CAD build for the part. Positions are in the model's coordinates, mm. Face numbers are marked on the shaded views. Round coordinates to 2 decimals unless told otherwise and drop trailing zeros. Order: outer loops, then holes, each group sorted by start corner. A loop starts at its lowest first (then second) coordinate and runs counter-clockwise, first axis right, second up. Notation, with made-up numbers: M -8,10.5 L 8,10.5 A11 ccw 8,25.5 Z; hole C 68.5,-24 d3. An arc over 180 degrees is marked long. Put each result on its own line as item: value.
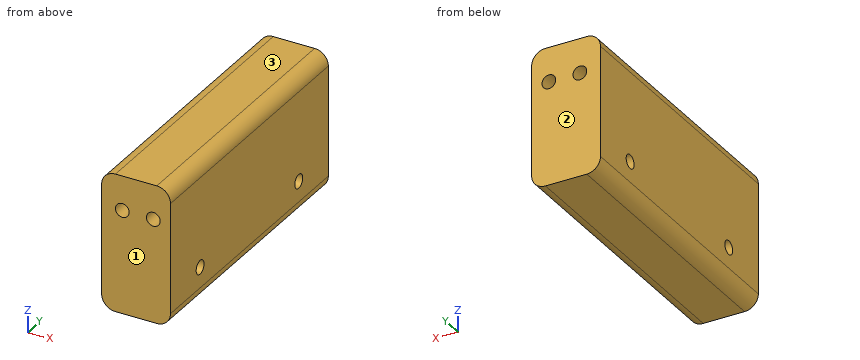
```python
from build123d import *

# Parameters (mm, degrees)
CYLINDER054_R       = 2
CYLINDER054_DEPTH   = 100
ARRAY001031_Y_COUNT = 2
ARRAY001031_Y_PITCH = 50
CYLINDER052_R       = 2
CYLINDER052_DEPTH   = 100
ARRAY001030_X_COUNT = 2
ARRAY001030_X_PITCH = 9
BOX029_W            = 20
BOX029_H            = 80
BOX029_DEPTH        = 40
FILLET001_R         = 4


with BuildPart() as horizontal_hole_array005:
    # Cylinder054 → Cylinder054 (new body)
    with BuildSketch(Plane(origin=(-50, 15, -10), x_dir=(0, 0, -1), z_dir=(1, 0, 0))):
        Circle(CYLINDER054_R)
    extrude(amount=CYLINDER054_DEPTH)

    # Array001031 Y: horizontal hole array005 ×2


with BuildPart() as horizontal_hole_array005_1:
    add(horizontal_hole_array005.part)
    with Locations(*[(0, i * ARRAY001031_Y_PITCH, 0) for i in range(1, ARRAY001031_Y_COUNT)]):
        add(horizontal_hole_array005.part)


with BuildPart() as stand_attachment_hole_fusion002:
    # Cylinder052 → Cylinder052 (new body)
    with BuildSketch(Plane(origin=(0, -10, 10), x_dir=(1, 0, 0), z_dir=(0, 1, 0))):
        Circle(CYLINDER052_R)
    extrude(amount=CYLINDER052_DEPTH)

    # Array001030 X: stand attachment hole fusion002 ×2


with BuildPart() as stand_attachment_hole_fusion002_1:
    add(stand_attachment_hole_fusion002.part)
    with Locations(*[(i * ARRAY001030_X_PITCH, 0, 0) for i in range(1, ARRAY001030_X_COUNT)]):
        add(stand_attachment_hole_fusion002.part)

    # Fusion025: union horizontal hole array005
    add(horizontal_hole_array005_1.part)


with BuildPart() as stand_attachment_middle_fillet001:
    # Box029 → Box029 (new body)
    with BuildSketch(Plane(origin=(-6, 0, -20), x_dir=(1, 0, 0), z_dir=(0, 0, 1))):
        with Locations((10, 40)):
            Rectangle(BOX029_W, BOX029_H)
    extrude(amount=BOX029_DEPTH)

    # Cut019004: cut stand attachment hole fusion002
    add(stand_attachment_hole_fusion002_1.part, mode=Mode.SUBTRACT)


with BuildPart() as stand_attachment_middle_fillet001_1:
    # Cut019004 placement: moved
    add(stand_attachment_middle_fillet001.part.moved(Location((-94, 0, -91))))

    # Fillet001
    fillet001_edges = [stand_attachment_middle_fillet001_1.edges().sort_by_distance(p)[0] for p in [
        (-100, 40, -71),
        (-100, 40, -111),
        (-80, 40, -71),
        (-80, 40, -111),
    ]]
    fillet(fillet001_edges, radius=FILLET001_R)


solid = stand_attachment_middle_fillet001_1.part
```
Item 1: Mould opens along Y. For the marked faces 1, 2 and 3 say: pulls with the +Y half, pulls with the -Y half, needs draft (parallel to the pull), parting line crosses it, or undercut.
Answers below:
face 1: pulls with the -Y half
face 2: pulls with the +Y half
face 3: needs draft
Item 2: Band-saw the part on B-B on y = 15. Give the cut face in (x, z), and give its area (3 significant figures).
Answers below:
outline: M -100,-107 A4 ccw -96,-111 L -84,-111 A4 ccw -80,-107 L -80,-103 L -100,-103 Z; M -100,-99 L -80,-99 L -80,-75 A4 ccw -84,-71 L -96,-71 A4 ccw -100,-75 Z; hole C -94,-81 d4; hole C -85,-81 d4
area: 681 mm²
Item 3: Band-saw the part on D-D on z = -101.5. Give the cut face in (x, y), and give its area (3 significant figures).
Answers below:
outline: M -100,0 L -80,0 L -80,13.06 L -100,13.06 Z; M -100,16.94 L -80,16.94 L -80,63.06 L -100,63.06 Z; M -100,66.94 L -80,66.94 L -80,80 L -100,80 Z
area: 1,450 mm²
Item 4: Probe line 1 along Y through (x, z) = (-85.5, -101); line 2 along X through (y, z) = (56, -81); line 3 along Z through (x, y) = (-85.25, 15). List the from-to ranges inside material, lowest first. Write a range as [from, to].
Answers below:
line 1: [0, 13], [17, 63], [67, 80]
line 2: [-100, -96], [-92, -87], [-83, -80]
line 3: [-111, -103], [-99, -82.98], [-79.02, -71]
Item 5: Band-saw the part on C-C on y = 62. Give the cut face in (x, z).
Answers below:
outline: M -100,-107 A4 ccw -96,-111 L -84,-111 A4 ccw -80,-107 L -80,-75 A4 ccw -84,-71 L -96,-71 A4 ccw -100,-75 Z; hole C -94,-81 d4; hole C -85,-81 d4
Item 6: Band-saw the part on A-A on x = -85. Give the cut face in (y, z), and give its area (3 significant figures).
Answers below:
outline: M 0,-111 L 80,-111 L 80,-83 L 0,-83 Z; M 0,-79 L 80,-79 L 80,-71 L 0,-71 Z; hole C 15,-101 d4; hole C 65,-101 d4
area: 2,850 mm²
Item 7: Pin check, flat tips, straight feed: P1, Ø2, axis at x = -82, y = 36, coming from the +Z side; P2, Ø3.5, axis at y = 65, z = -101, coming from the +X side. Stop position of each tip, or through.
Answers below:
P1: z = -71.13
P2: through
